```python
from build123d import *

# Parameters (mm, degrees)
BOSS_EXTRUDE1_DEPTH = 0.6
CUT_EXTRUDE1_DEPTH  = 2
SKETCH3_R           = 0.525
CUT_EXTRUDE2_DEPTH  = 10
BOSS_EXTRUDE2_DEPTH = 0.5
SKETCH5_R           = 2.5
BOSS_EXTRUDE3_DEPTH = 1.3
SKETCH6_R           = 2.5
SKETCH6_R_2         = 2.2
CUT_EXTRUDE3_DEPTH  = 0.2
FILLET1_R           = 1
CHAMFER1_SIZE       = 1


with BuildPart() as part:
    # Sketch1 → Boss-Extrude1 (new body)
    with BuildSketch(Plane(origin=(0, 0, 0), x_dir=(1, 0, 0), z_dir=(0, 1, 0))):
        with BuildLine():
            Line((-7.75, -13.25), (7.75, -13.25))
            ThreePointArc((7.75, -13.25), (9.871320344, -12.371320344), (10.75, -10.25))
            Line((10.75, -10.25), (10.75, 10.25))
            ThreePointArc((10.75, 10.25), (9.871320344, 12.371320344), (7.75, 13.25))
            Line((7.75, 13.25), (-7.75, 13.25))
            ThreePointArc((-7.75, 13.25), (-9.871320344, 12.371320344), (-10.75, 10.25))
            Line((-10.75, 10.25), (-10.75, -10.25))
            ThreePointArc((-10.75, -10.25), (-9.871320344, -12.371320344), (-7.75, -13.25))
        make_face()
    extrude(amount=BOSS_EXTRUDE1_DEPTH)

    # Sketch2 → Cut-Extrude1 (cut)
    with BuildSketch(Plane(origin=(0, 0.6, 0), x_dir=(1, 0, 0), z_dir=(0, 1, 0))):
        with BuildLine():
            Line((1.55, -10), (-8.05, -10))
            ThreePointArc((-8.05, -10), (-8.226776695, -9.926776695), (-8.3, -9.75))
            Line((-8.3, -9.75), (-8.3, -0.15))
            ThreePointArc((-8.3, -0.15), (-8.226776695, 0.026776695), (-8.05, 0.1))
            Line((-8.05, 0.1), (1.55, 0.1))
            ThreePointArc((1.55, 0.1), (1.726776695, 0.026776695), (1.8, -0.15))
            Line((1.8, -0.15), (1.8, -9.75))
            ThreePointArc((1.8, -9.75), (1.726776695, -9.926776695), (1.55, -10))
        make_face()
    extrude(amount=-CUT_EXTRUDE1_DEPTH, mode=Mode.SUBTRACT)

    # Sketch3 → Cut-Extrude2 (cut)
    with BuildSketch(Plane(origin=(0, 0.6, 0), x_dir=(1, 0, 0), z_dir=(0, 1, 0))):
        with Locations((-8.05, -2.35)):
            Circle(SKETCH3_R)
        Polygon((2.2, -6.969264593), (2.2, -8.531138717), (1.8, -8.867190969), (1.8, -6.633227233), align=None)
    extrude(amount=-CUT_EXTRUDE2_DEPTH, mode=Mode.SUBTRACT)

    # Sketch4 → Boss-Extrude2 (add)
    with BuildSketch(Plane(origin=(0, 0, 0), x_dir=(-1, 0, 0), z_dir=(0, -1, 0))):
        with BuildLine():
            Line((7.75, 12.25), (-7.75, 12.25))
            ThreePointArc((-7.75, 12.25), (-9.164213562, 11.664213562), (-9.75, 10.25))
            Line((-9.75, 10.25), (-9.75, -10.25))
            ThreePointArc((-9.75, -10.25), (-9.164213562, -11.664213562), (-7.75, -12.25))
            Line((-7.75, -12.25), (7.75, -12.25))
            ThreePointArc((7.75, -12.25), (9.164213562, -11.664213562), (9.75, -10.25))
            Line((9.75, -10.25), (9.75, 10.25))
            ThreePointArc((9.75, 10.25), (9.164213562, 11.664213562), (7.75, 12.25))
        make_face()
        with BuildLine():
            Line((7.75, 11.5), (-7.75, 11.5))
            ThreePointArc((-7.75, 11.5), (-8.633883476, 11.133883476), (-9, 10.25))
            Line((-9, 10.25), (-9, -10.25))
            ThreePointArc((-9, -10.25), (-8.633883476, -11.133883476), (-7.75, -11.5))
            Line((-7.75, -11.5), (7.75, -11.5))
            ThreePointArc((7.75, -11.5), (8.633883476, -11.133883476), (9, -10.25))
            Line((9, -10.25), (9, 10.25))
            ThreePointArc((9, 10.25), (8.633883476, 11.133883476), (7.75, 11.5))
        make_face(mode=Mode.SUBTRACT)
    extrude(amount=BOSS_EXTRUDE2_DEPTH)

    # Sketch5 → Boss-Extrude3 (add)
    with BuildSketch(Plane(origin=(0, 0, 0), x_dir=(-1, 0, 0), z_dir=(0, -1, 0))):
        with Locations(Location((-4.25, 4.45, 0), (0, 0, 90))):
            Circle(SKETCH5_R)
        with Locations(Location((4.25, 4.45, 0), (0, 0, 90))):
            Circle(SKETCH5_R)
    extrude(amount=BOSS_EXTRUDE3_DEPTH)

    # Sketch6 → Cut-Extrude3 (cut)
    # profile 1 of 2: a face of its own
    with BuildSketch(Plane(origin=(0, 0.6, 0), x_dir=(1, 0, 0), z_dir=(0, 1, 0))):
        with Locations(Location((4.25, 4.45, 0), (0, 0, 90))):
            Circle(SKETCH6_R)
        with Locations(Location((4.25, 4.45, 0), (0, 0, 270))):
            Circle(SKETCH6_R_2, mode=Mode.SUBTRACT)
    # profile 2 of 2: a face of its own
    with BuildSketch(Plane(origin=(0, 0.6, 0), x_dir=(1, 0, 0), z_dir=(0, 1, 0))):
        with Locations(Location((-4.25, 4.45, 0), (0, 0, 90))):
            Circle(SKETCH6_R)
        with Locations(Location((-4.25, 4.45, 0), (0, 0, 270))):
            Circle(SKETCH6_R_2, mode=Mode.SUBTRACT)
    extrude(amount=-CUT_EXTRUDE3_DEPTH, mode=Mode.SUBTRACT)

    # Fillet1
    # the kernel refuses this fillet: 1 mm, written as the material it takes off along each edge
    with BuildSketch(Plane(origin=(4.25, 0.6, -4.45), x_dir=(0, 0, -1), z_dir=(1, 0, 0))) as fillet1_piece_1:
        with BuildLine():
            CenterArc((3.1, -1), FILLET1_R, 90, 36.869897646)
            Line((2.5, -0.2), (2.488, -0.184))
            ThreePointArc((2.488, -0.184), (2.48, -0.1), (2.48, 0))
            Line((2.48, 0), (2.5, 0.02))
            Line((2.5, 0.02), (3.1, 0.02))
            Line((3.1, 0.02), (3.1, 0))
        make_face()
    revolve(axis=Axis((4.25, 0.6, -4.45), (0, 1, 0)), mode=Mode.SUBTRACT)
    with BuildSketch(Plane(origin=(4.25, 0.6, -4.45), x_dir=(0, 0, 1), z_dir=(-1, 0, 0))) as fillet1_piece_2:
        with BuildLine():
            CenterArc((1.6, -1), FILLET1_R, 53.130102354, 36.869897646)
            Line((1.6, 0), (1.6, 0.02))
            Line((1.6, 0.02), (2.2, 0.02))
            Line((2.2, 0.02), (2.22, 0))
            ThreePointArc((2.22, 0), (2.22, -0.1), (2.212, -0.184))
            Line((2.212, -0.184), (2.2, -0.2))
        make_face()
    revolve(axis=Axis((4.25, 0.6, -4.45), (0, 1, 0)), mode=Mode.SUBTRACT)
    with BuildSketch(Plane(origin=(-4.25, 0.6, -4.45), x_dir=(0, 0, -1), z_dir=(1, 0, 0))) as fillet1_piece_3:
        with BuildLine():
            CenterArc((3.1, -1), FILLET1_R, 90, 36.869897646)
            Line((2.5, -0.2), (2.488, -0.184))
            ThreePointArc((2.488, -0.184), (2.48, -0.1), (2.48, 0))
            Line((2.48, 0), (2.5, 0.02))
            Line((2.5, 0.02), (3.1, 0.02))
            Line((3.1, 0.02), (3.1, 0))
        make_face()
    revolve(axis=Axis((-4.25, 0.6, -4.45), (0, 1, 0)), mode=Mode.SUBTRACT)
    with BuildSketch(Plane(origin=(-4.25, 0.6, -4.45), x_dir=(0, 0, 1), z_dir=(-1, 0, 0))) as fillet1_piece_4:
        with BuildLine():
            CenterArc((1.6, -1), FILLET1_R, 53.130102354, 36.869897646)
            Line((1.6, 0), (1.6, 0.02))
            Line((1.6, 0.02), (2.2, 0.02))
            Line((2.2, 0.02), (2.22, 0))
            ThreePointArc((2.22, 0), (2.22, -0.1), (2.212, -0.184))
            Line((2.212, -0.184), (2.2, -0.2))
        make_face()
    revolve(axis=Axis((-4.25, 0.6, -4.45), (0, 1, 0)), mode=Mode.SUBTRACT)

    # Chamfer1
    chamfer1_edges = [part.edges().sort_by_distance(p)[0] for p in [
        (4.25, -1.3, -1.95),
        (-4.25, -1.3, -1.95),
    ]]
    chamfer(chamfer1_edges, length=CHAMFER1_SIZE)


solid = part.part
```
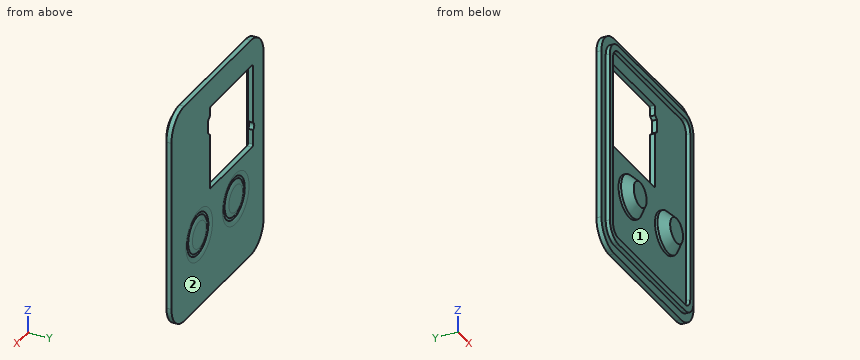
Work out the finished part from the listing and answer in its coordinate system (mm). Face numbers are marked on the shaded views. Coordinates: 2 decimals unless noted, no trailing zeros. Write each loop counter-clockwise with the first axis right and the second up, starting at its lowest first coordinate (ties: lowest second). Pieces come first, ordered by that corner, then holes. Notation, with made-up numbers: (8, 68) - (52, 68) arc R6 ccw to (52, 72) - close; hole circle Ø6 at (-32, 1.25). An arc over 180 degrees is marked (long way). Answer as a JSON object with one key per item and string values.
Q1. For a pull along Z with two mould halves and no side action, classify the marked faces 1 and 2 as pulls with the +Z half, pulls with the -Z half, needs draft (parallel to the pull), parting line crosses it, or undercut.
Results list:
{"face 1": "undercut", "face 2": "needs draft"}
Q2. Find section C-C (y = -0.8). Write down the section's boundary in (x, z), plus the area to 3 significant figures.
Results list:
{"outline": "circle Ø4 at (-4.25, -4.45); circle Ø4 at (4.25, -4.45)", "area": "25.1 mm^2"}
Q3. Consider L1, parallel to X at y = -0.35, z = 5.5; L2, parallel to X at y = 0.25, z = 0.75; L3, parallel to Y at x = -9.5, z = -4.25. Determine where each line is inside the solid, lowest interval first. Write a range as from..to.
Results list:
{"L1": "x = -9.75..-9, 9..9.75", "L2": "x = -10.75..-8.3, 1.8..10.75", "L3": "y = -0.5..0.6"}
Q4. Find section A-A (z = 5.5). Write down the section's boundary in (x, y).
Results list:
{"outline": "(-10.75, 0) - (-9.75, 0) - (-9.75, -0.5) - (-9, -0.5) - (-9, 0) - (-8.3, 0) - (-8.3, 0.6) - (-10.75, 0.6) - close; (1.8, 0) - (9, 0) - (9, -0.5) - (9.75, -0.5) - (9.75, 0) - (10.75, 0) - (10.75, 0.6) - (1.8, 0.6) - close"}
Q5. Find section B-B (x = 4.25). Write down the section's boundary in (y, z).
Results list:
{"outline": "(-1.3, -5.95) - (-0.3, -6.95) - (0, -6.95) - (0, -11.5) - (-0.5, -11.5) - (-0.5, -12.25) - (0, -12.25) - (0, -13.25) - (0.6, -13.25) - (0.6, -7.55) arc R1 ccw to (0.4, -6.95) - (0.4, -6.65) arc R1 ccw to (0.6, -6.05) - (0.6, -2.85) arc R1 ccw to (0.4, -2.25) - (0.4, -1.95) arc R1 ccw to (0.6, -1.35) - (0.6, 13.25) - (0, 13.25) - (0, 12.25) - (-0.5, 12.25) - (-0.5, 11.5) - (0, 11.5) - (0, -1.95) - (-0.3, -1.95) - (-1.3, -2.95) - close"}
Q6. Given pin 1 Ø0.6 at (y, z) = (-0.5, 1) entering from +X; pin 2 Ø6.5 at (x, z) = (-0.5, 4.5) entering from -Y, each flat-ended and moving along its own axis, determine where each tip first touches the part or whether it passes through.
Results list:
{"pin 1": "stops at x = 9.75", "pin 2": "stops at y = 0"}
